Source: CAD feature listing. Evaluate the final solid. Frame: model axes, mm. Face numbers are marked on the shaded views. Give positions to 0.01 mm unless a question says otherwise; leave off trailing zeros. Order: outer loops, then holes, each group sorted by start corner. A loop starts at its lowest first (then second) coordinate and runs counter-clockwise, first axis right, second up. Notation, with made-up numbers: (43, -34) - (67, -34) arc R27 ccw to (67, -11) - close; hole circle Ø9 at (22, 8.25). An arc over 180 degrees is marked (long way). One line per item, written item: value. Start each with the question number.
from build123d import *

# Parameters (mm, degrees)
CONG_1_R = 4
CONG_2_R = 0.5
CONG_4_R = 1


with BuildPart() as part:
    # Esquisse1 → Révolution1 (revolve)
    with BuildSketch(Plane.XY, mode=Mode.PRIVATE) as r_volution1_sk:
        Polygon((-8.23, 14.28840181), (-14.48, 14.28840181), (-14.48, 12.18840181), (-10.48, 12.18840181), (-10.48, 9.78840181), (-7.75, 7.88840181), (-6.75, 3.88840181), (-4.4, 3.88840181), (-5.25, 11.28840181), align=None)
    revolve(r_volution1_sk.sketch.rotate(Axis((0, 31.998542825, 0), (0, -1, 0)), 270), axis=Axis((0, 31.998542825, 0), (0, -1, 0)))  # turned: the seam where the file's is

    # Congé1
    cong_1_edges = [part.edges().sort_by_distance(p)[0] for p in [
        (0, 7.88840181, -7.75),
    ]]
    fillet(cong_1_edges, radius=CONG_1_R)

    # Congé2
    cong_2_edges = [part.edges().sort_by_distance(p)[0] for p in [
        (0, 3.88840181, -4.4),
    ]]
    fillet(cong_2_edges, radius=CONG_2_R)

    # Congé4
    cong_4_edges = [part.edges().sort_by_distance(p)[0] for p in [
        (0, 14.28840181, -14.48),
    ]]
    fillet(cong_4_edges, radius=CONG_4_R)


solid = part.part
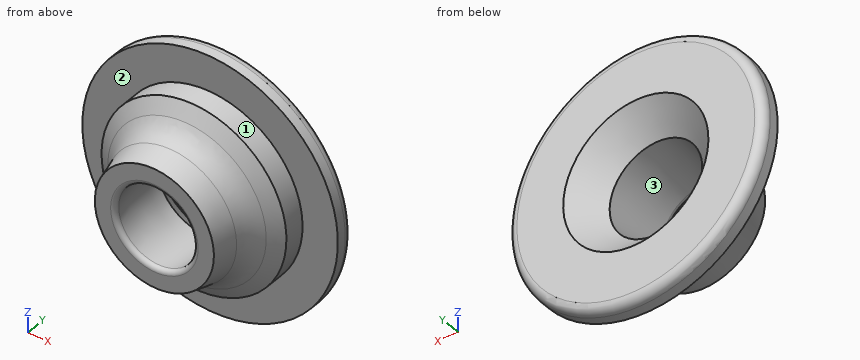
1. Ray query, L1, parallel to Y at x = -0.5, z = -11.25; L2, parallel to X at y = 12.25, z = 4.5; L3, parallel to X at y = 6.25, z = -1.5. Return the intervals inside material, ascending.
2. Section A-A on y = 13.75. Return the cut outline in (x, z), then the cut area to 3 significant figures.
3. Section B-B on y = 10.75. Return the cut outline in (x, z), then the cut area to 3 significant figures.
4. Contact query for flat-ended pins moving along their axis: pin 1 Ø3 at (y, z) = (8.5, 8) entering from +X; pin 2 Ø6 at (y, z) = (11.5, -8.5) entering from -X. Output: stop coordinate, or through.
5. Draft query along Z for the marked faces 1, 2 and 3. Return one class per face: pulls with the +Z half, pulls with the -Z half, needs draft (parallel to the pull), parting line crosses it, or undercut.
Data:
1. L1: y = 12.19 to 14.29
1. L2: x = -13.76 to -4.27, 4.27 to 13.76
1. L3: x = -7.19 to -4.42, 4.42 to 7.19
2. outline: circle Ø28.73 at (0, 0); hole circle Ø15.39 at (0, 0)
2. area: 462 mm2
3. outline: circle Ø20.96 at (0, 0); hole circle Ø10.38 at (0, 0)
3. area: 260 mm2
4. pin 1: stops at x = 7.58
4. pin 2: stops at x = -13.36
5. face 1: parting line crosses it
5. face 2: needs draft
5. face 3: undercut
